Geometry: see drawing. Coordinates: mm, zero at the bounding-box minimum. A direction names the side the tool comes from. Coordinates: 2 decimals unless noted, no trailing zeros. Order: outer loops, then holes, each group sorted by start corner. A loop starts at its lowest first (then second) coordinate and runs counter-clockwise, first axis right, second up. Notation, with made-up numbers: (80, 53.5) - (105, 53.5) arc R6 ccw to (105, 59.5) - close; hole circle Ø7 at (27, -32). An arc over 180 degrees is marked (long way). Use a Markdown table: item, result. Add a question column.
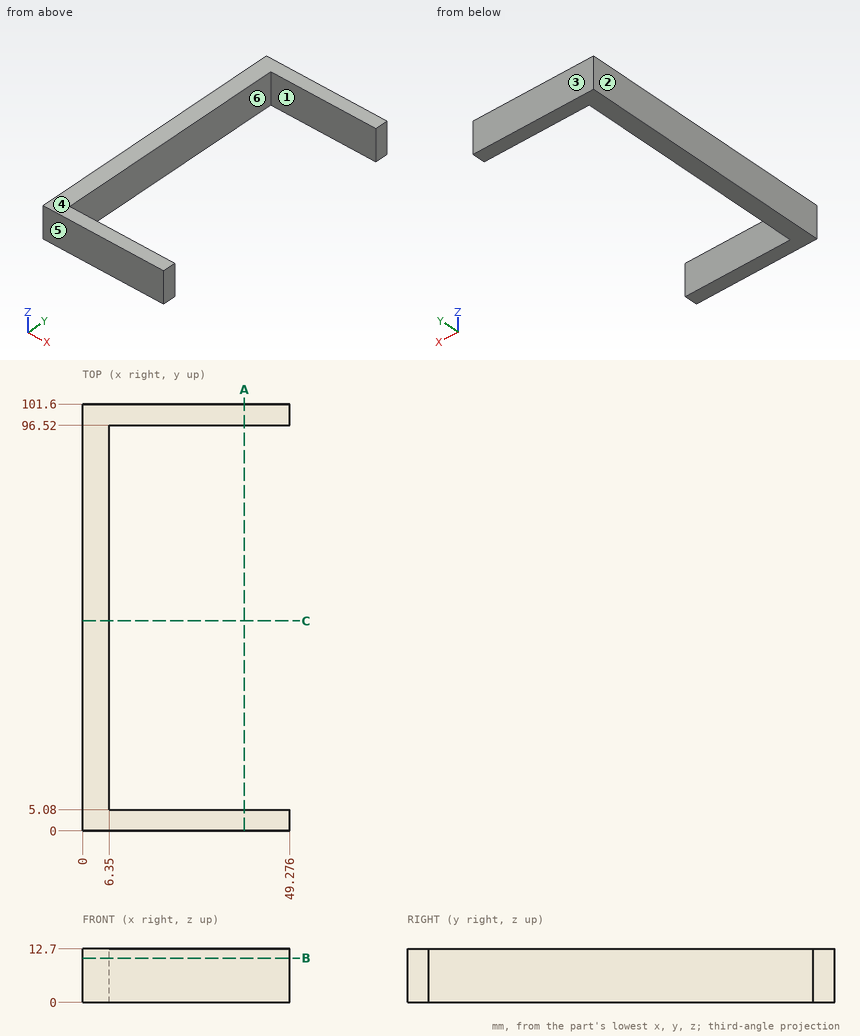
1) Draft query along Y for the marked faces 3, 4, 5 and 6. Return one class per face: released by +Y, released by -Y, zero draft, split by the parting line, or undercut.
2) Access query for the marked faces 1 and 2. Directions: +Z, -Z, +X, -X, +Y, -Y. A direction counts if a zero-diameter tool reaches every point of the face in a straight line with its end or side. Return the directions, or none.
3) Section query B-B (z = 10.5). Return the cut outline in (x, y), and give its area (3 significant figures).
4) Section query A-A (x = 38.5). Return the cut outline in (y, z).
5) Section query C-C (y = 50). Return the cut outline in (x, z), and give its area (3 significant figures).
6) Line query: line 1 (Y direction, x = 33, z = 6.75); line 2 (X direction, y = 19, z = 11.25). Output: solid intervals per line, ascending. Write a range as from..to.
From the geometry:
| question | item | result |
|---|---|---|
| 1 | face 3 | released by +Y |
| 1 | face 4 | zero draft |
| 1 | face 5 | released by -Y |
| 1 | face 6 | undercut |
| 2 | face 1 | +Z, -Z, +X |
| 2 | face 2 | +Z, -Z, -X, +Y, -Y |
| 3 | outline | (0, 0) - (49.28, 0) - (49.28, 5.08) - (6.35, 5.08) - (6.35, 96.52) - (49.28, 96.52) - (49.28, 101.6) - (0, 101.6) - close |
| 3 | area | 1,080 mm^2 |
| 4 | outline | (0, 0) - (5.08, 0) - (5.08, 12.7) - (0, 12.7) - close; (96.52, 0) - (101.6, 0) - (101.6, 12.7) - (96.52, 12.7) - close |
| 5 | outline | (0, 0) - (6.35, 0) - (6.35, 12.7) - (0, 12.7) - close |
| 5 | area | 80.6 mm^2 |
| 6 | line 1 | y = 0..5.08, 96.52..101.6 |
| 6 | line 2 | x = 0..6.35 |
